Geometry: final body of the model. Coordinates: model frame, mm. Face numbers are marked on the shaded views. A direction names the side the tool comes from. Round coordinates to 2 decimals unless told otherwise and drop trailing zeros. Order: outer loops, then holes, each group sorted by start corner. A loop starts at its lowest first (then second) coordinate and runs counter-clockwise, first axis right, second up. Notation, with made-up numbers: M 5.25,60.5 L 45.25,60.5 A13 cw 45.25,68.5 Z; hole C 56,83 d3. An arc over 180 degrees is marked long. Put each result on its own line as item: value. Start each with the question number.
1) Access query for the marked faces 4, 5, 6, 7 and 8. Directions: +Z, -Z, +X, -X, +Y, -Y. A direction counts if a zero-diameter tool reaches every point of the face in a straight line with its end or side. Return the directions, or none.
2) Section B-B, the plane x = 0.25. Return loops of the section in (y, z), then the cut area to 3 significant figures.
3) Section C-C, the plane y = -2.5. Return loops of the section in (x, z).
4) First-contact query: P1, Ø1, axis at x = 8, y = -6.5, coming from the -Z side. Flat tip, straight axial feed; report the tip coordinate or a pass-through.
5) Material intervals for probe 1 along X at (y, z) = (6.25, 0.95); probe 2 along Y at (x, z) = (-5.75, 0.15); probe 3 along X at (y, z) = (5.25, 0.2), sorted ascending. Write a range as [from, to].
6) Draft query along Y for the marked faces 1, 2 and 3. Return one class per face: pulls with the +Y half, pulls with the -Y half, needs draft (parallel to the pull), parting line crosses it, or undercut.
7) Section D-D, the plane y = -9. Return loops of the section in (x, z).
from build123d import *

# Parameters (mm, degrees)
F1_DEPTH = 2
F2_T     = -1.5
F3_SIZE  = 0.4


with BuildPart() as f1:
    # F0 (on Top) → F1 (new body)
    with BuildSketch(Plane.XY):
        Polygon((0, 10.5), (-2.0710678119, 5), (-7.4246212025, 7.4246212025), (-5, 2.0710678119), (-10.5, 0), (-5, -2.0710678119), (-7.4246212025, -7.4246212025), (-2.0710678119, -5), (0, -10.5), (2.0710678119, -5), (7.4246212025, -7.4246212025), (5, -2.0710678119), (10.5, 0), (5, 2.0710678119), (7.4246212025, 7.4246212025), (2.0710678119, 5), align=None)
    extrude(amount=F1_DEPTH)

    # F2
    f2_openings = [f1.faces().sort_by_distance(p)[0] for p in [
        (0, 0, 2),
    ]]
    offset(amount=F2_T, openings=f2_openings, kind=Kind.INTERSECTION)

    # F3
    f3_edges = [f1.edges().sort_by_distance(p)[0] for p in [
        (6.212311, -4.747845, 0),
        (7.75, -1.035534, 0),
        (7.75, 1.035534, 0),
        (6.212311, 4.747845, 0),
        (4.747845, 6.212311, 0),
        (1.035534, 7.75, 0),
        (-1.035534, 7.75, 0),
        (-4.747845, 6.212311, 0),
        (-6.212311, 4.747845, 0),
        (-7.75, 1.035534, 0),
        (-7.75, -1.035534, 0),
        (-6.212311, -4.747845, 0),
        (-4.747845, -6.212311, 0),
        (-1.035534, -7.75, 0),
        (1.035534, -7.75, 0),
        (4.747845, -6.212311, 0),
    ]]
    chamfer(f3_edges, length=F3_SIZE)


solid = f1.part
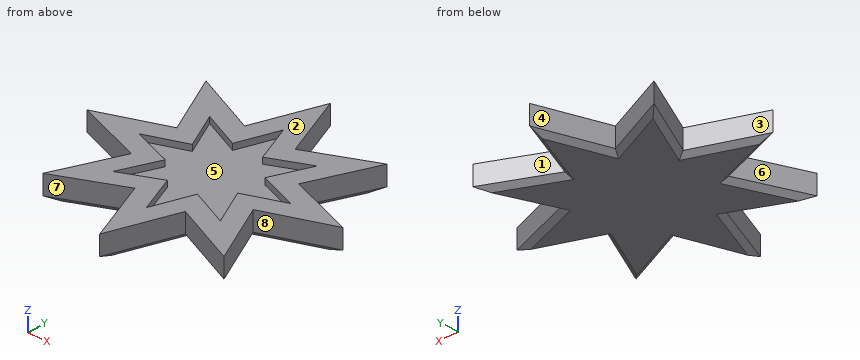
Result sheet:
1. face 4: +Z, -Z, +Y
1. face 5: +Z
1. face 6: +Z, -Z, -X
1. face 7: +Z, -Z, -Y
1. face 8: +Z, -Z, +X
2. outline: M -9.84,0.4 L -8.7,0 L 8.7,0 L 9.84,0.4 L 9.84,2 L 5.58,2 L 5.58,1.5 L -5.58,1.5 L -5.58,2 L -9.84,2 Z
2. area: 33.3 mm2
3. outline: M -5.19,0.4 L -4.76,0 L 4.76,0 L 5.19,0.4 L 5.19,2 L 3.55,2 L 3.55,1.5 L -3.55,1.5 L -3.55,2 L -5.19,2 Z
4. P1: passes through
5. probe 1: x = [-6.89, -4.83], [-1.6, 1.6], [4.83, 6.89]
5. probe 2: y = [-6.39, -4.33], [-1.52, 1.52], [4.33, 6.39]
5. probe 3: x = [-6.22, -3.11], [-1.76, 1.76], [3.11, 6.22]
6. face 1: pulls with the +Y half
6. face 2: needs draft
6. face 3: undercut
7. outline: M -0.56,0.4 L -0.14,0 L 0.14,0 L 0.56,0.4 L 0.56,2 L -0.56,2 Z
